```python
from build123d import *

# Parameters (mm, degrees)
F0_R     = 5.5
F1_DEPTH = 8
F2_R     = 5.5
F3_DEPTH = 50


with BuildPart() as f1:
    # F0 (on Front) → F1 (new body)
    with BuildSketch(Plane.XZ):
        Polygon((8.660254, 5), (0, 10), (-8.660254, 5), (-8.660254, -5), (0, -10), (8.660254, -5), align=None)
        Circle(F0_R, mode=Mode.SUBTRACT)
    extrude(amount=-F1_DEPTH)

    # F2 (on Front) → F3 (join)
    with BuildSketch(Plane.XZ):
        Circle(F2_R)
    extrude(amount=-F3_DEPTH)


solid = f1.part
```
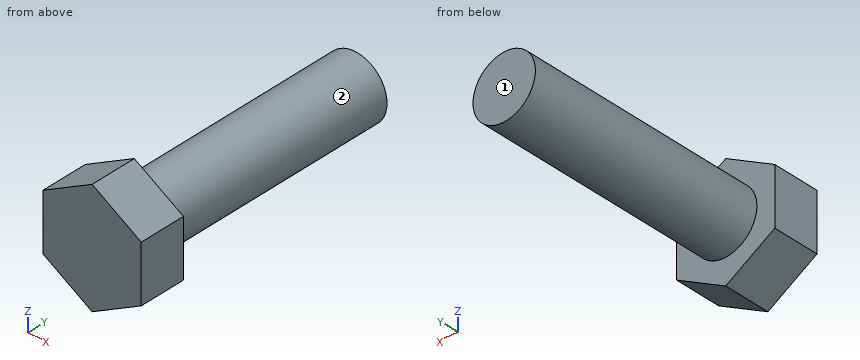
Verification items for the finished model (mm, model axes). Face numbers are marked on the shaded views. A direction names the side the tool comes from. Coordinates: 2 decimals unless noted, no trailing zeros. Order: outer loops, then holes, each group sorted by start corner. A loop starts at its lowest first (then second) coordinate and runs counter-clockwise, first axis right, second up. Notation, with made-up numbers: (18.25, 62.25) - (51.25, 62.25) arc R13 cw to (51.25, 85.25) - close; hole circle Ø5 at (80.25, 10). An arc over 180 degrees is marked (long way). Return JSON: item names as keys, results as strings.
(1) Section check D-D, the plane x = -6.5. Record the cut outline in (y, z).
Filled sheet:
{"outline": "(0, -6.25) - (8, -6.25) - (8, 6.25) - (0, 6.25) - close"}
(2) Section check C-C, the plane z = 2. Record the cut outline in (x, y), and give its area (3 significant figures).
Filled sheet:
{"outline": "(-8.66, 0) - (8.66, 0) - (8.66, 8) - (5.12, 8) - (5.12, 50) - (-5.12, 50) - (-5.12, 8) - (-8.66, 8) - close", "area": "569 mm^2"}
(3) Thickness scan on line 1 along Y through (x, z) = (-2.5, -7); line 2 along Z through (x, y) = (4.75, 42); line 3 along Z through (x, y) = (-1.5, 29). Record the ranges inside material, lowest first.
Filled sheet:
{"line 1": "y = 0 to 8", "line 2": "z = -2.77 to 2.77", "line 3": "z = -5.29 to 5.29"}
(4) Section check A-A, the plane z = 0. Record the cut outline in (x, y), and give its area (3 significant figures).
Filled sheet:
{"outline": "(-8.66, 0) - (8.66, 0) - (8.66, 8) - (5.5, 8) - (5.5, 50) - (-5.5, 50) - (-5.5, 8) - (-8.66, 8) - close", "area": "601 mm^2"}
(5) Access from +Z, -Z, +X, -X, +Y, -Y to the whole of each face (thin tool, end or side, straight path). Record for the marked faces 1 and 2.
Filled sheet:
{"face 1": "+Z, -Z, +X, -X, +Y", "face 2": "+Y"}
(6) Go/stop test with flat-tipped pins: pin 1 (10 mm diameter, centred on y = 13.5, z = -3, fed in from +X); pin 2 (1.5 mm diameter, centred on x = 1, y = 21.5, fed in from -Z); pin 3 (10 mm diameter, centred on x = -2, z = -0.5, fed in from -Y); pin 4 (6 mm diameter, centred on x = -4, y = 17, fed in from -Z). Record where each tip stops, or that it passes through.
Filled sheet:
{"pin 1": "stops at x = 5.5", "pin 2": "stops at z = -5.49", "pin 3": "stops at y = 0", "pin 4": "stops at z = -5.41"}
(7) Section check B-B, the plane y = 10.5. Record the cut outline in (x, z).
Filled sheet:
{"outline": "circle Ø11 at (0, 0)"}
